Build history of the part. All positions in model axes, mm. A direction names the side the tool comes from. Give positions to 0.01 mm unless a question says otherwise; leave off trailing zeros. Order: outer loops, then holes, each group sorted by start corner. A loop starts at its lowest first (then second) coordinate and runs counter-clockwise, first axis right, second up. Notation, with made-up numbers: M 49.5,48 L 98.5,48 A33 ccw 98.5,77 Z; hole C 47,63.25 d6. An arc over 180 degrees is marked long. Answer as CSV lines item,"result".
from build123d import *

# Parameters (mm, degrees)
SKETCH1_W                                      = 190
SKETCH1_H                                      = 10
BOSS_EXTRUDE1_DEPTH                            = 5
SKETCH2_W                                      = 185.9
SKETCH2_H                                      = 4.99
BOSS_EXTRUDE2_DEPTH                            = 205
CBORE_FOR_M3_SOCKET_HEAD_CAP_SCREW1_AT_2_COUNT = 2
CBORE_FOR_M3_SOCKET_HEAD_CAP_SCREW1_AT_2_PITCH = 176
CBORE_FOR_M3_SOCKET_HEAD_CAP_SCREW1_AT_3_COUNT = 2
CBORE_FOR_M3_SOCKET_HEAD_CAP_SCREW1_AT_3_PITCH = 258.940147524
CBORE_FOR_M3_SOCKET_HEAD_CAP_SCREW1_AT_4_COUNT = 2
CBORE_FOR_M3_SOCKET_HEAD_CAP_SCREW1_AT_4_PITCH = 189
SKETCH6_W                                      = 190
SKETCH6_H                                      = 22.149014811
CUT_EXTRUDE1_DEPTH                             = 10


with BuildPart() as part:
    # Sketch1 → Boss-Extrude1 (new body)
    with BuildSketch(Plane.XY):
        Rectangle(SKETCH1_W, SKETCH1_H)
    extrude(amount=BOSS_EXTRUDE1_DEPTH)

    # Sketch2 → Boss-Extrude2 (add)
    with BuildSketch(Plane(origin=(0, 0, 0), x_dir=(-1, 0, 0), z_dir=(0, 0, -1))):
        Rectangle(SKETCH2_W, SKETCH2_H)
    extrude(amount=BOSS_EXTRUDE2_DEPTH)

    # Sketch5 → CBORE for M3 Socket Head Cap Screw1 (revolve, cut)
    with BuildSketch(Plane(origin=(-87.95, 2.495, -7), x_dir=(0, 0, 1), z_dir=(1, 0, 0))):
        Polygon((0, 0), (0, 21.081549114), (1.8, 20), (1.8, 3.4), (3.25, 3.4), (3.25, 0.025), (3.275, 0), align=None)
    cbore_for_m3_socket_head_cap_screw1 = revolve(axis=Axis((-87.95, 8.845, -7), (0, -1, 0)), mode=Mode.SUBTRACT)

    # CBORE for M3 Socket Head Cap Screw1 at 2: CBORE for M3 Socket Head Cap Screw1 ×2
    with Locations(*[(i * CBORE_FOR_M3_SOCKET_HEAD_CAP_SCREW1_AT_2_PITCH, 0, 0) for i in range(1, CBORE_FOR_M3_SOCKET_HEAD_CAP_SCREW1_AT_2_COUNT)]):
        add(cbore_for_m3_socket_head_cap_screw1, mode=Mode.SUBTRACT)

    # CBORE for M3 Socket Head Cap Screw1 at 3: CBORE for M3 Socket Head Cap Screw1 ×2
    with Locations(*[Vector(0.683555647, 0, -0.729898402) * (i * CBORE_FOR_M3_SOCKET_HEAD_CAP_SCREW1_AT_3_PITCH) for i in range(1, CBORE_FOR_M3_SOCKET_HEAD_CAP_SCREW1_AT_3_COUNT)]):
        add(cbore_for_m3_socket_head_cap_screw1, mode=Mode.SUBTRACT)

    # CBORE for M3 Socket Head Cap Screw1 at 4: CBORE for M3 Socket Head Cap Screw1 ×2
    with Locations(*[(0, 0, -i * CBORE_FOR_M3_SOCKET_HEAD_CAP_SCREW1_AT_4_PITCH) for i in range(1, CBORE_FOR_M3_SOCKET_HEAD_CAP_SCREW1_AT_4_COUNT)]):
        add(cbore_for_m3_socket_head_cap_screw1, mode=Mode.SUBTRACT)

    # Sketch6 → Cut-Extrude1 (cut)
    with BuildSketch(Plane(origin=(0, 0, 0), x_dir=(-1, 0, 0), z_dir=(0, 0, -1))):
        with Locations((0, -13.569507406)):
            Rectangle(SKETCH6_W, SKETCH6_H)
    extrude(amount=-CUT_EXTRUDE1_DEPTH, mode=Mode.SUBTRACT)


solid = part.part
Item 1: Band-saw the part on A-A (y = 1.25). Give the cut face in (x, z).
Geometry says:
outline,"M -95,0 L -92.95,0 L -92.95,-205 L 92.95,-205 L 92.95,0 L 95,0 L 95,5 L -95,5 Z; hole C -87.95,-196 d6.5; hole C -87.95,-7 d6.5; hole C 88.05,-7 d6.5; hole C 89.05,-196 d6.5"
Item 2: Probe line 1 along X through (y, z) = (0.4, -7); line 2 along Z through (x, y) = (88.05, 1.7); line 3 along X through (y, z) = (-1.15, -196). List the from-to ranges inside material, lowest first. Write a range as from..to.
Geometry says:
line 1,"x = -92.95..-91.2, -84.7..84.8, 91.3..92.95"
line 2,"z = -205..-199.09, -192.91..-10.25, -3.75..5"
line 3,"x = -92.95..-89.75, -86.15..87.25, 90.85..92.95"
Item 3: Drop flat-ended pins along their axis: pin 1 (4 mm diameter, centred on x = 88.05, z = -7, fed in from -Y) (3 decimals); pin 2 (4 mm diameter, centred on y = -1, z = -81, fed in from -X); pin 3 (7 mm diameter, centred on x = 87.5, z = -196.5, fed in from +Y) (3 decimals); pin 4 (2 mm diameter, centred on x = -89, z = -6, fed in from +Y) (3 decimals). Give the stop position or say it passes through.
Geometry says:
pin 1,"stops at y = -2.495"
pin 2,"stops at x = -92.95"
pin 3,"stops at y = 2.495"
pin 4,"stops at y = -0.905"
Item 4: Band-saw the part on C-C (z = -99). Give the cut face in (x, y) (3 decimals), and give its area (3 significant figures).
Geometry says:
outline,"M -92.95,-2.495 L 92.95,-2.495 L 92.95,2.495 L -92.95,2.495 Z"
area,"928 mm2"
Item 5: Pull direction X, two halves, no side cores. Call faces 4 (the flat face through (-1, 1, 5)), 5 (the flat face through (-86.55, -0.905, -197.4)), 6 (the flat face through (92.95, 0, -101)): released by +X, released by -X, zero draft, split by the parting line, or undercut.
Geometry says:
face 4,"zero draft"
face 5,"undercut"
face 6,"released by +X"
Item 6: 3-axis set-ups, long thin cutter, end or side, ignore diameter. For faces 1 (the flat face through (1, 2.495, -101)), 2 (the flat face through (-92.95, 0, -101)), 3 (the cylindrical face through (90.3, 0.8, -193)): which of +Z, -Z, +X, -X, +Y, -Y reach the whole face in a straight line?
Geometry says:
face 1,"-Z, +X, -X, +Y"
face 2,"-Z, -X, +Y, -Y"
face 3,"+Y"
Item 7: Band-saw the part on B-B (x = -34). Give the cut face in (y, z) (3 decimals), and give its area (3 significant figures).
Geometry says:
outline,"M -2.495,-205 L 2.495,-205 L 2.495,0 L 5,0 L 5,5 L -2.495,5 Z"
area,"1,060 mm2"
